Geometry check sheet. Reference: the model listing, model coordinates, mm. Face numbers are marked on the shaded views. A direction names the side the tool comes from. Round coordinates to 2 decimals unless told otherwise and drop trailing zeros. Order: outer loops, then holes, each group sorted by start corner. A loop starts at its lowest first (then second) coordinate and runs counter-clockwise, first axis right, second up.
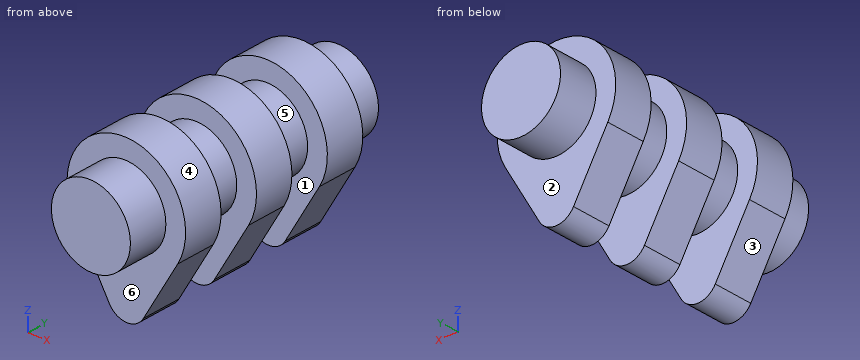
```python
from build123d import *

# Parameters (mm, degrees)
F0_R      = 12.7
F1_DEPTH  = 88.9
F3_R      = 12.7
F4_DEPTH  = 12.7
F6_R      = 12.7
F7_DEPTH  = 12.7
F9_R      = 12.7
F10_DEPTH = 12.7


with BuildPart() as f1:
    # F0 (on Front) → F1 (new body)
    with BuildSketch(Plane.XZ):
        Circle(F0_R)
    extrude(amount=F1_DEPTH)

    # F3 (on offset) → F4 (join)
    with BuildSketch(Plane.XZ.offset(12.7)):
        with BuildLine():
            Line((5.499261, -28.575), (16.497784, -9.525))
            ThreePointArc((16.497784, -9.525), (0, 19.05), (-16.497784, -9.525))
            Line((-16.497784, -9.525), (-5.499261, -28.575))
            ThreePointArc((-5.499261, -28.575), (0, -31.75), (5.499261, -28.575))
        make_face()
        Circle(F3_R, mode=Mode.SUBTRACT)
    extrude(amount=F4_DEPTH)

    # F6 (on offset) → F7 (join)
    with BuildSketch(Plane.XZ.offset(38.1)):
        with BuildLine():
            Line((5.499261, -28.575), (16.497784, -9.525))
            ThreePointArc((16.497784, -9.525), (0, 19.05), (-16.497784, -9.525))
            Line((-16.497784, -9.525), (-5.499261, -28.575))
            ThreePointArc((-5.499261, -28.575), (0, -31.75), (5.499261, -28.575))
        make_face()
        Circle(F6_R, mode=Mode.SUBTRACT)
    extrude(amount=F7_DEPTH)

    # F9 (on offset) → F10 (join)
    with BuildSketch(Plane.XZ.offset(63.5)):
        with BuildLine():
            Line((5.499261, -28.575), (16.497784, -9.525))
            ThreePointArc((16.497784, -9.525), (0, 19.05), (-16.497784, -9.525))
            Line((-16.497784, -9.525), (-5.499261, -28.575))
            ThreePointArc((-5.499261, -28.575), (0, -31.75), (5.499261, -28.575))
        make_face()
        Circle(F9_R, mode=Mode.SUBTRACT)
    extrude(amount=F10_DEPTH)


solid = f1.part
```
(1) Set-up check for the marked faces 4, 5 and 6: record each of +Z, -Z, +X, -X, +Y, -Y from which the full face is reachable in a straight line by a thin tool's end or side.
Returned:
face 4: +Y, -Y
face 5: none
face 6: -Y
(2) Sectioned sample at D-D, the plane y = -69.5. Record the cut outline in (x, z) (3 decimals).
Returned:
outline: (-16.498, -9.525) - (-5.499, -28.575) arc R6.35 ccw to (5.499, -28.575) - (16.498, -9.525) arc R19.05 ccw (long way) to start
(3) Sectioned sample at C-C, the plane y = -10. Record the cut outline in (x, z).
Returned:
outline: circle Ø25.4 at (0, 0)
(4) Sectioned sample at B-B, the plane z = 0. Record the cut outline in (x, y).
Returned:
outline: (-19.05, -76.2) - (-12.7, -76.2) - (-12.7, -88.9) - (12.7, -88.9) - (12.7, -76.2) - (19.05, -76.2) - (19.05, -63.5) - (12.7, -63.5) - (12.7, -50.8) - (19.05, -50.8) - (19.05, -38.1) - (12.7, -38.1) - (12.7, -25.4) - (19.05, -25.4) - (19.05, -12.7) - (12.7, -12.7) - (12.7, 0) - (-12.7, 0) - (-12.7, -12.7) - (-19.05, -12.7) - (-19.05, -25.4) - (-12.7, -25.4) - (-12.7, -38.1) - (-19.05, -38.1) - (-19.05, -50.8) - (-12.7, -50.8) - (-12.7, -63.5) - (-19.05, -63.5) - close
(5) Sectioned sample at A-A, the plane x = 0. Record the cut outline in (y, z).
Returned:
outline: (-88.9, -12.7) - (-76.2, -12.7) - (-76.2, -31.75) - (-63.5, -31.75) - (-63.5, -12.7) - (-50.8, -12.7) - (-50.8, -31.75) - (-38.1, -31.75) - (-38.1, -12.7) - (-25.4, -12.7) - (-25.4, -31.75) - (-12.7, -31.75) - (-12.7, -12.7) - (0, -12.7) - (0, 12.7) - (-12.7, 12.7) - (-12.7, 19.05) - (-25.4, 19.05) - (-25.4, 12.7) - (-38.1, 12.7) - (-38.1, 19.05) - (-50.8, 19.05) - (-50.8, 12.7) - (-63.5, 12.7) - (-63.5, 19.05) - (-76.2, 19.05) - (-76.2, 12.7) - (-88.9, 12.7) - close
(6) Material ranges on line 1 (Y direction, x = 2.5, z = -18.5); line 2 (X direction, y = -69, z = 0.5); line 3 (Z direction, x = 4.5, y = -5), recorded low to high.
Returned:
line 1: y = -76.2 to -63.5, -50.8 to -38.1, -25.4 to -12.7
line 2: x = -19.04 to 19.04
line 3: z = -11.88 to 11.88
(7) Draft check along Y on the marked faces 1, 2 and 3. Enter one of: released by +Y, released by -Y, zero draft, split by the parting line, or undercut.
Returned:
face 1: undercut
face 2: released by +Y
face 3: zero draft
(8) Depth check by flat-ended pin: P1, Ø11.5, axis at x = 5, z = -17.5, coming from the -Y side; P2, Ø3, axis at x = 12.5, y = -53, coming from the +Z side; P3, Ø6, axis at y = -68, z = -5, coming from the +X side; P4, Ø5, axis at x = -0.5, y = -55.5, coming from the +Z side. Enter the tip coordinate at first touch or a pass-through.
Returned:
P1: stops at y = -88.9
P2: stops at z = 6.35
P3: stops at x = 18.94
P4: stops at z = 12.7
